Check sheet for the modelled part. Datum: model origin and axes. Units: mm. A direction names the side the tool comes from. Round coordinates to 2 decimals unless told otherwise and drop trailing zeros. Order: outer loops, then holes, each group sorted by start corner. A loop starts at its lowest first (then second) coordinate and runs counter-clockwise, first axis right, second up.
Q1. Depth check by flat-ended pin: P1, Ø3, axis at x = 7.5, z = -3.5, coming from the +Y side; P2, Ø2, axis at x = 11.5, z = 3.5, coming from the +Y side; P3, Ø1, axis at x = -0.5, y = -2, coming from the +Z side. Enter the tip coordinate at first touch or a pass-through.
Q2. Set-up check for faces 4 (the cylindrical face through (-12.57, 4.05, 2.58)), 5 (the cylindrical face through (-13.82, -3.03, 3.95)): record each of +Z, -Z, +X, -X, +Y, -Y from which the full face is reachable in a straight line by a thin tool's end or side.
Q3. Cross-section at A-A on x = 7. Record the cut outline in (y, z), then the cut area to 3 significant figures.
Q4. Scan lines: probe 1 along Y at (x, z) = (9.75, -0.25); probe 2 along Y at (x, z) = (-1.25, -2); probe 3 along Z at (x, y) = (0.25, -1). Record each from-to range of solid material in increasing order.
Q5. Mould release check, pull along X, two halves, no side actions. Record for faces 1 (the flat face through (15, 0, 0)), 2 (the cylindrical face through (12.57, 4.05, 2.58)), 3 (the cylindrical face through (0.17, -3.03, 3.95)): +X half, -X half, draft (parallel to the pull), parting line (faces both ways), or undercut.
from build123d import *

# Parameters (mm, degrees)
SKETCH1_R           = 4.98
BOSS_EXTRUDE1_DEPTH = 15
CUT_EXTRUDE1_START  = -3
SKETCH2_R           = 4.98
SKETCH2_R_2         = 4.8
CUT_EXTRUDE1_DEPTH  = 1.15
CHAMFER1_SIZE       = 0.5
CHAMFER2_SIZE       = 0.5


with BuildPart() as part:
    # Sketch1 → Boss-Extrude1 (new, symmetric)
    with BuildSketch(Plane(origin=(0, 0, 0), x_dir=(0, 0, -1), z_dir=(1, 0, 0))):
        Circle(SKETCH1_R)
    extrude(amount=BOSS_EXTRUDE1_DEPTH, both=True)

    # Sketch2 → Cut-Extrude1 (cut)
    with BuildSketch(Plane.ZY.offset(15).offset(CUT_EXTRUDE1_START)):
        Circle(SKETCH2_R)
        Circle(SKETCH2_R_2, mode=Mode.SUBTRACT)
    cut_extrude1 = extrude(amount=CUT_EXTRUDE1_DEPTH, mode=Mode.SUBTRACT)

    # Chamfer1
    chamfer1_edges = [part.edges().sort_by_distance(p)[0] for p in [
        (-15, 0, 4.98),
    ]]
    chamfer(chamfer1_edges, length=CHAMFER1_SIZE)

    # Mirror1: Cut-Extrude1 across plane
    add(cut_extrude1.mirror(Plane(origin=(0, 0, 0), x_dir=(0, 0, 1), z_dir=(1, 0, 0))), mode=Mode.SUBTRACT)

    # Chamfer2
    chamfer2_edges = [part.edges().sort_by_distance(p)[0] for p in [
        (15, 0, 4.98),
    ]]
    chamfer(chamfer2_edges, length=CHAMFER2_SIZE)


solid = part.part
Results found:
1. P1: stops at y = 4.56
1. P2: stops at y = 4.31
1. P3: stops at z = 4.75
2. face 4: none
2. face 5: +X, -X
3. outline: circle Ø9.96 at (0, 0)
3. area: 77.9 mm2
4. probe 1: y = -4.97 to 4.97
4. probe 2: y = -4.56 to 4.56
4. probe 3: z = -4.88 to 4.88
5. face 1: +X half
5. face 2: undercut
5. face 3: draft
